Read the model definition and answer for the solid it produces. Units are mm, in the model's axes. A direction names the side the tool comes from. Round coordinates to 2 decimals unless told otherwise and drop trailing zeros. Write each loop counter-clockwise with the first axis right and the second up, starting at its lowest first coordinate (ties: lowest second). Pieces come first, ordered by that corner, then holes. Notation, with made-up numbers: (80.25, 53) -> (92.25, 53) arc R12 ccw to (92.25, 76) -> close; hole circle Ø2 at (72.25, -40). An arc over 180 degrees is marked (long way). Return JSON: item names as keys, results as strings. Group by question number.
(1) A cutting plane is placed at A-A on x = 0. Give the vertices of the cut face in (y, z).
(2) A cutting plane is placed at D-D on x = 5.75. Give the vertices of the cut face in (y, z), then the cut area to 3 significant figures.
(3) For faces 4 (the cylindrical face through (-1.08, -4.88, 8.43)), 5 (the cylindrical face through (-1.08, -4.88, -0.76)), 6 (the cylindrical face through (-0.867, -3.905, 5.895)), determine the directions among +Z, -Z, +X, -X, +Y, -Y from which every point of the face is accessible in a straight line to the end or side of a thin tool.
(4) The mould has two halves that part along X. Classify faces 1 (the flat face through (2, -5, 3.5)), 2 (the cylindrical face through (-2.396, -10.789, 1.726)), 3 (the cylindrical face through (-3.694, -8.166, 1.726)): released by +X, released by -X, zero draft, split by the parting line, or undercut.
(5) Given pin 1 (2 mm diameter, centred on x = -6.5, y = -7, fed in from +Z); pin 2 (1 mm diameter, centred on y = 5, z = 9.5, fed in from +X); pin 3 (1.5 mm diameter, centred on x = 5.5, y = 3, fed in from -Z); pin 4 (2 mm diameter, centred on x = 4.5, y = 6.61, fed in from -Z), each flat-ended and moving along its own axis, determine where each tip first touches the part or whether it passes through.
(6) A cutting plane is placed at C-C on z = 10.5. Give the vertices of the cut face in (x, y).
(7) Straight lines are drawn through the part: line 1 (Y direction, x = -2, z = 9); line 2 (X direction, y = -6.75, z = 2); line 3 (Z direction, x = 0, y = 6). For each, find the intervals that lie inside material, in ascending order.
```python
from build123d import *

# Parameters (mm, degrees)
SKETCH_1_R           = 11.051525353
SKETCH_1_R_2         = 5
SKETCH_1_R_3         = 1.75
EXTRUDE_2_DEPTH      = 3.5
EXTRUDE_3_DEPTH      = 13.5
EXTRUDE_3_DEPTH_BACK = 1.5
SKETCH_1_5_R         = 5
SKETCH_1_5_R_2       = 4


with BuildPart() as part:
    # Sketch 1 → Extrude 2 (new body)
    with BuildSketch(Plane.XY):
        Circle(SKETCH_1_R)
        Circle(SKETCH_1_R_2, mode=Mode.SUBTRACT)
        with Locations((6.613016892, -4.502000398)):
            Circle(SKETCH_1_R_3, mode=Mode.SUBTRACT)
        with Locations((4.502000398, 6.613016892)):
            Circle(SKETCH_1_R_3, mode=Mode.SUBTRACT)
        with Locations((-6.613016892, 4.502000398)):
            Circle(SKETCH_1_R_3, mode=Mode.SUBTRACT)
        with Locations((-4.502000398, -6.613016892)):
            Circle(SKETCH_1_R_3, mode=Mode.SUBTRACT)
    extrude(amount=EXTRUDE_2_DEPTH)

    # Sketch 1_5 → Extrude 3 (add, two sides: drawn at the far end of the back side and taken through both)
    with BuildSketch(Plane.XY.offset(-EXTRUDE_3_DEPTH_BACK)):
        Circle(SKETCH_1_5_R)
        Circle(SKETCH_1_5_R_2, mode=Mode.SUBTRACT)
    extrude(amount=EXTRUDE_3_DEPTH + EXTRUDE_3_DEPTH_BACK)


solid = part.part
```
Checks:
{
 "1": {"outline": "(-11.05, 0) -> (-5, 0) -> (-5, -1.5) -> (-4, -1.5) -> (-4, 13.5) -> (-5, 13.5) -> (-5, 3.5) -> (-11.05, 3.5) -> close; (4, -1.5) -> (5, -1.5) -> (5, 0) -> (11.05, 0) -> (11.05, 3.5) -> (5, 3.5) -> (5, 13.5) -> (4, 13.5) -> close"},
 "2": {"outline": "(-9.44, 0) -> (-6.02, 0) -> (-6.02, 3.5) -> (-9.44, 3.5) -> close; (-2.98, 0) -> (5.39, 0) -> (5.39, 3.5) -> (-2.98, 3.5) -> close; (7.84, 0) -> (9.44, 0) -> (9.44, 3.5) -> (7.84, 3.5) -> close", "area": "46.8 mm^2"},
 "3": {"face 4": "+Z", "face 5": "-Z", "face 6": "+Z, -Z"},
 "4": {"face 1": "zero draft", "face 2": "split by the parting line", "face 3": "undercut"},
 "5": {"pin 1": "stops at z = 3.5", "pin 2": "stops at x = 2.18", "pin 3": "stops at z = 0", "pin 4": "passes through"},
 "6": {"outline": "circle Ø10 at (0, 0); hole circle Ø8 at (0, 0)"},
 "7": {"line 1": "y = -4.58 to -3.46, 3.46 to 4.58", "line 2": "x = -8.75 to -6.25, -2.76 to 8.75", "line 3": "z = 0 to 3.5"}
}
